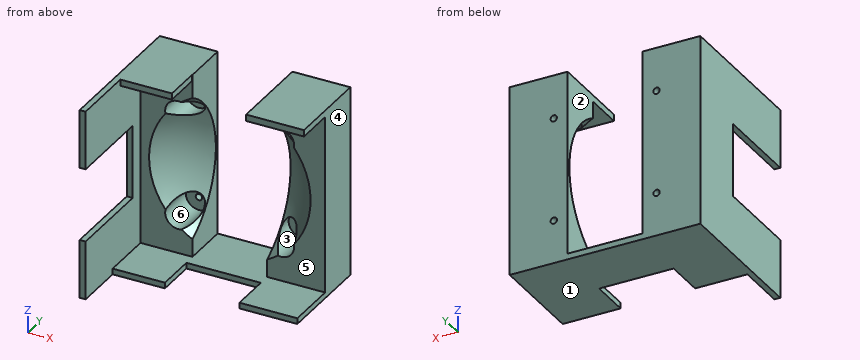
from build123d import *
from build123d.topology import SkipClean

# Parameters (mm, degrees)
SKETCH1_W                   = 102
SKETCH1_H                   = 102
BOSS_EXTRUDE1_DEPTH         = 50
CUT_EXTRUDE_THIN1_OUTLINE_W = 40
CUT_EXTRUDE_THIN1_OUTLINE_H = 95.773670058
CUT_EXTRUDE_THIN1_DEPTH     = 50
SKETCH4_W                   = 40
SKETCH4_H                   = 6.202657501
CUT_EXTRUDE3_DEPTH          = 54
SKETCH5_W                   = 33.817621941
SKETCH5_H                   = 102.594578927
CUT_EXTRUDE4_DEPTH          = 20
SKETCH6_W                   = 27.820383201
SKETCH6_H                   = 98.886835029
CUT_EXTRUDE5_DEPTH          = 20
SKETCH7_W                   = 30.8
SKETCH7_H                   = 3.364819678
BOSS_EXTRUDE2_DEPTH         = 21
SKETCH9_W                   = 31
SKETCH9_H                   = 3.479961613
BOSS_EXTRUDE4_DEPTH         = 21
SKETCH11_W                  = 98.820383201
SKETCH11_H                  = 3.113164971
BOSS_EXTRUDE6_DEPTH         = 47.625
SKETCH14_W                  = 102
SKETCH14_H                  = 5
CUT_EXTRUDE7_DEPTH          = 105
SKETCH17_R                  = 7
CUT_EXTRUDE12_DEPTH         = 20.5
M3_CLEARANCE_HOLE1_D        = 3.4
SKETCH22_W                  = 3.179616799
SKETCH22_H                  = 102
BOSS_EXTRUDE7_DEPTH         = 47.6
SKETCH23_W                  = 98.820383201
SKETCH23_H                  = 3.113164971
CUT_EXTRUDE13_DEPTH         = 40
SKETCH24_W                  = 102
SKETCH24_H                  = 13.144479163
CUT_EXTRUDE14_DEPTH         = 10
SKETCH25_W                  = 39.837829701
SKETCH25_H                  = 21.316982849
CUT_EXTRUDE15_DEPTH         = 6
SKETCH26_W                  = 39.22350869
SKETCH26_H                  = 46.778434415
CUT_EXTRUDE16_DEPTH         = 6


# Read off the part's stored shape, not the designer's step: Cut-Extrude-Thin1
with BuildPart() as part:
    # Sketch1 → Boss-Extrude1 (new body)
    with BuildSketch(Plane(origin=(0, 0, 0), x_dir=(1, 0, 0), z_dir=(0, 1, 0))):
        with Locations((-66.567363259, 25.977216604)):
            Rectangle(SKETCH1_W, SKETCH1_H)
    extrude(amount=BOSS_EXTRUDE1_DEPTH)

    # Sketch2 → Cut-Revolve1 (revolve, cut)
    with SkipClean():  # the faces are left unmerged after this step: merging them gives an invalid solid
        with BuildSketch(Plane(origin=(0, 0, 0), x_dir=(1, 0, 0), z_dir=(0, 1, 0))):
            with BuildLine():
                ThreePointArc((-66.567363259, 73.602216604), (-114.192363259, 25.977216604), (-66.567363259, -21.647783396))
                Line((-66.567363259, -21.647783396), (-66.567363259, 73.602216604))
            make_face()
            with BuildLine():
                Line((-66.567363259, 73.602216604), (-66.567363259, -21.647783396))
                ThreePointArc((-66.567363259, -21.647783396), (-32.891402805, -7.69874385), (-18.942363259, 25.977216604))
                ThreePointArc((-18.942363259, 25.977216604), (-32.891402805, 59.653177058), (-66.567363259, 73.602216604))
            make_face()
        revolve(axis=Axis((-66.567363259, 0, 21.647783396), (0, 0, -1)), mode=Mode.SUBTRACT)
    add(part.part.scale(1), mode=Mode.REPLACE)  # the faces are merged on a copy

    # Cut-Extrude-Thin1 outline → Cut-Extrude-Thin1 (cut)
    with BuildSketch(Plane(origin=(0, 0, 0), x_dir=(1, 0, 0), z_dir=(0, 1, 0))):
        with Locations((-66.567363259, 25.977216604)):
            Rectangle(CUT_EXTRUDE_THIN1_OUTLINE_W, CUT_EXTRUDE_THIN1_OUTLINE_H)
    extrude(amount=CUT_EXTRUDE_THIN1_DEPTH, mode=Mode.SUBTRACT)

    # Sketch4 → Cut-Extrude3 (cut)
    with BuildSketch(Plane(origin=(0, 0, 0), x_dir=(1, 0, 0), z_dir=(0, 1, 0))):
        with Locations((-66.567363259, -25.010947176)):
            Rectangle(SKETCH4_W, SKETCH4_H)
    extrude(amount=CUT_EXTRUDE3_DEPTH, mode=Mode.SUBTRACT)

    # Sketch5 → Cut-Extrude4 (cut)
    with BuildSketch(Plane(origin=(0, 0, 0), x_dir=(1, 0, 0), z_dir=(0, 1, 0))):
        with Locations((-29.658552289, 22.56676217)):
            Rectangle(SKETCH5_W, SKETCH5_H)
    extrude(amount=CUT_EXTRUDE4_DEPTH, mode=Mode.SUBTRACT)

    # Sketch6 → Cut-Extrude5 (cut)
    with BuildSketch(Plane(origin=(0, 0, 0), x_dir=(-1, 0, 0), z_dir=(0, -1, 0))):
        with Locations((100.47755486, 24.420634119)):
            Rectangle(SKETCH6_W, SKETCH6_H)
    extrude(amount=-CUT_EXTRUDE5_DEPTH, mode=Mode.SUBTRACT)

    # Sketch7 → Boss-Extrude2 (add)
    with BuildSketch(Plane(origin=(0, 0, 0), x_dir=(1, 0, 0), z_dir=(0, 1, 0))):
        with Locations((-102.167363259, -23.340373557)):
            Rectangle(SKETCH7_W, SKETCH7_H)
    extrude(amount=BOSS_EXTRUDE2_DEPTH)

    # Sketch9 → Boss-Extrude4 (add)
    with BuildSketch(Plane.XZ.offset(-20)):
        with Locations((-31.067363259, 23.28280259)):
            Rectangle(SKETCH9_W, SKETCH9_H)
    extrude(amount=BOSS_EXTRUDE4_DEPTH)

    # Sketch11 → Boss-Extrude6 (add)
    with BuildSketch(Plane.XZ):
        with Locations((-64.97755486, -75.420634119)):
            Rectangle(SKETCH11_W, SKETCH11_H)
    extrude(amount=BOSS_EXTRUDE6_DEPTH)

    # Sketch14 → Cut-Extrude7 (cut)
    with BuildSketch(Plane(origin=(-15.567363259, 0, 0), x_dir=(0, 0, -1), z_dir=(1, 0, 0))):
        with Locations((25.977216604, 47.5)):
            Rectangle(SKETCH14_W, SKETCH14_H)
    extrude(amount=-CUT_EXTRUDE7_DEPTH, mode=Mode.SUBTRACT)

    # Sketch17 → Cut-Extrude12 (cut)
    with BuildSketch(Plane.XZ.offset(-20)):
        with Locations(Location((-94.167363259, 1.657963718, 0), (0, 0, 270))):
            Circle(SKETCH17_R)
        with Locations(Location((-94.167363259, -53.864051633, 0), (0, 0, 284.685382437))):
            Circle(SKETCH17_R)
        with Locations(Location((-39.167363259, 1.657963718, 0), (0, 0, 349.246729183))):
            Circle(SKETCH17_R)
        with Locations(Location((-39.167363259, -53.864051633, 0), (0, 0, 270))):
            Circle(SKETCH17_R)
    extrude(amount=-CUT_EXTRUDE12_DEPTH, mode=Mode.SUBTRACT)

    # M3 Clearance Hole1 (through all)
    with Locations(Plane(origin=(0, 40.5, 0), x_dir=(-1, 0, 0), z_dir=(0, -1, 0))):
        with Locations((94.167363259, -1.657963718), (39.167363259, -1.657963718), (39.167363259, 53.864051633), (94.167363259, 53.864051633)):
            Hole(M3_CLEARANCE_HOLE1_D / 2)

    # Sketch22 → Boss-Extrude7 (add)
    with BuildSketch(Plane.XZ):
        with Locations((-115.97755486, -25.977216604)):
            Rectangle(SKETCH22_W, SKETCH22_H)
    extrude(amount=BOSS_EXTRUDE7_DEPTH)

    # Sketch23 → Cut-Extrude13 (cut)
    with BuildSketch(Plane.XZ.offset(47.625)):
        with Locations((-64.97755486, -75.420634119)):
            Rectangle(SKETCH23_W, SKETCH23_H)
    extrude(amount=-CUT_EXTRUDE13_DEPTH, mode=Mode.SUBTRACT)

    # Sketch24 → Cut-Extrude14 (cut)
    with BuildSketch(Plane(origin=(-114.38774646, 0, 0), x_dir=(0, 0, -1), z_dir=(1, 0, 0))):
        with Locations((25.977216604, -41.027760419)):
            Rectangle(SKETCH24_W, SKETCH24_H)
    extrude(amount=-CUT_EXTRUDE14_DEPTH, mode=Mode.SUBTRACT)

    # Sketch25 → Cut-Extrude15 (cut)
    with BuildSketch(Plane.XY.offset(-73.864051633)):
        with Locations((-66.48627811, 3.033491424)):
            Rectangle(SKETCH25_W, SKETCH25_H)
    extrude(amount=-CUT_EXTRUDE15_DEPTH, mode=Mode.SUBTRACT)

    # Sketch26 → Cut-Extrude16 (cut)
    with BuildSketch(Plane(origin=(-114.38774646, 0, 0), x_dir=(0, 0, -1), z_dir=(1, 0, 0))):
        with Locations((25.942998987, -11.06630363)):
            Rectangle(SKETCH26_W, SKETCH26_H)
    extrude(amount=-CUT_EXTRUDE16_DEPTH, mode=Mode.SUBTRACT)


solid = part.part
Input: part model. Units: mm. Frame: model coordinates. Face numbers are marked on the shaded views. A direction names the side the tool comes from. Round coordinates to 2 decimals unless told otherwise and drop trailing zeros. Order: outer loops, then holes, each group sorted by start corner. A loop starts at its lowest first (then second) coordinate and runs counter-clockwise, first axis right, second up. Notation, with made-up numbers: (18.5, 73) - (71.5, 73) arc R14 cw to (71.5, 98) - close; hole circle Ø1 at (5, -33.5). An arc over 180 degrees is marked (long way). Use a Markdown table: item, result.
1. Section B-B on y = 6.5. Return the cut outline in (x, z), then the cut area to 3 significant figures.
Evaluation:
| item | result |
|---|---|
| outline | (-117.57, -76.98) - (-86.41, -76.98) - (-86.41, -73.86) - (-114.39, -73.86) - (-114.39, -45.55) - (-117.57, -45.55) - close; (-117.57, -6.33) - (-114.39, -6.33) - (-114.39, 21.66) - (-86.77, 21.66) - (-86.77, 25.02) - (-117.57, 25.02) - close; (-46.57, -76.98) - (-15.57, -76.98) - (-15.57, -73.86) - (-46.57, -73.86) - close; (-46.57, 21.54) - (-15.57, 21.54) - (-15.57, 25.02) - (-46.57, 25.02) - close |
| area | 584 mm^2 |
2. Section D-D on z = -14.5. Return the cut outline in (x, y), then the cut area to 3 significant figures.
Evaluation:
| item | result |
|---|---|
| outline | (-117.57, 12.32) - (-114.39, 12.32) - (-114.39, 20) - (-108.24, 20) arc R46.22 cw to (-86.57, 41.67) - (-86.57, 45) - (-117.57, 45) - close; (-46.57, 41.67) arc R46.22 cw to (-24.9, 20) - (-15.57, 20) - (-15.57, 45) - (-46.57, 45) - close |
| area | 997 mm^2 |
3. Material intervals for probe 1 along Z at (x, y) = (-34, 18); probe 2 along Z at (x, y) = (-89, 16.5); probe 3 along X at (y, z) = (5, 20), sorted ascending.
Evaluation:
| item | result |
|---|---|
| probe 1 | -76.98 to -73.86, 21.54 to 25.02 |
| probe 2 | -76.98 to -73.86, 21.66 to 25.02 |
| probe 3 | -117.57 to -114.39 |
4. Mould query, pull axis X, two halves, no side actions, for the marked faces 4, 5 and 6. Classes: +X half, -X half, draft (parallel to the pull), parting line (faces both ways), or undercut.
Evaluation:
| item | result |
|---|---|
| face 4 | +X half |
| face 5 | draft |
| face 6 | undercut |
5. Access query for the marked faces 1, 2 and 3. Directions: +Z, -Z, +X, -X, +Y, -Y. A direction counts if a zero-diameter tool reaches every point of the face in a straight line with its end or side. Return the directions, or none.
Evaluation:
| item | result |
|---|---|
| face 1 | -Z, +X, -X, +Y, -Y |
| face 2 | +Z, +Y, -Y |
| face 3 | -Y |
6. Section C-C on y = 18. Return the cut outline in (x, z), then the cut area to 3 significant figures.
Evaluation:
| item | result |
|---|---|
| outline | (-117.57, -76.98) - (-15.57, -76.98) - (-15.57, -73.86) - (-114.39, -73.86) - (-114.39, 21.66) - (-86.77, 21.66) - (-86.77, 25.02) - (-117.57, 25.02) - close; (-46.57, 21.54) - (-15.57, 21.54) - (-15.57, 25.02) - (-46.57, 25.02) - close |
| area | 833 mm^2 |
7. Section A-A on y = -2.5. Return the cut outline in (x, z), then the cut area to 3 significant figures.
Evaluation:
| item | result |
|---|---|
| outline | (-117.57, -76.98) - (-86.41, -76.98) - (-86.41, -73.86) - (-114.39, -73.86) - (-114.39, -45.55) - (-117.57, -45.55) - close; (-117.57, -6.33) - (-114.39, -6.33) - (-114.39, 25.02) - (-117.57, 25.02) - close; (-46.57, -76.98) - (-15.57, -76.98) - (-15.57, -73.86) - (-46.57, -73.86) - close |
| area | 383 mm^2 |
8. First-contact query: pin 1 (6 mm diameter, centred on x = -26, z = -21.5, fed in from -Y); pin 2 (1 mm diameter, centred on y = 3, z = 8, fed in from +X); pin 3 (7 mm diameter, centred on x = -92, z = -53.5, fed in from -Y); pin 4 (2 mm diameter, centred on x = -94.17, z = -53.86, fed in from -Y). Flat tips, straight axial feed; report the tip coordinate or a pass-through.
Evaluation:
| item | result |
|---|---|
| pin 1 | y = 20 |
| pin 2 | x = -114.39 |
| pin 3 | y = 40.5 |
| pin 4 | through |
